from build123d import *

# Parameters (mm, degrees)
SKETCH1_W               = 52
SKETCH1_H               = 107
SKETCH1_R               = 3.25
BOSS_EXTRUDE1_DEPTH     = 3
SKETCH2_W               = 3
SKETCH2_H               = 35
BOSS_EXTRUDE2_DEPTH     = 35
SKETCH3_W               = 52
SKETCH3_H               = 5
BOSS_EXTRUDE3_DEPTH     = 25
SKETCH4_R               = 7.5
CUT_EXTRUDE1_DEPTH      = 71.585055075
CUT_EXTRUDE2_DEPTH      = 111.927904515
CUT_EXTRUDE2_DEPTH_BACK = 111.927904515
SKETCH5_W               = 35
SKETCH5_H               = 7


with BuildPart() as part:
    # Sketch1 → Boss-Extrude1 (new body)
    with BuildSketch(Plane(origin=(0, 0, 0), x_dir=(1, 0, 0), z_dir=(0, 1, 0))):
        Rectangle(SKETCH1_W, SKETCH1_H)
        with Locations(Location((17.5, -12, 0), (0, 0, 270))):
            Circle(SKETCH1_R, mode=Mode.SUBTRACT)
    extrude(amount=BOSS_EXTRUDE1_DEPTH)

    # Sketch2 → Boss-Extrude2 (add)
    with BuildSketch(Plane.XZ):
        with Locations((-24.5, 0)):
            Rectangle(SKETCH2_W, SKETCH2_H)
        with Locations((24.5, 0)):
            Rectangle(SKETCH2_W, SKETCH2_H)
    extrude(amount=BOSS_EXTRUDE2_DEPTH)

    # Sketch3 → Boss-Extrude3 (add)
    with BuildSketch(Plane.XZ):
        with Locations((0, 46)):
            Rectangle(SKETCH3_W, SKETCH3_H)
        with Locations((0, -46)):
            Rectangle(SKETCH3_W, SKETCH3_H)
    extrude(amount=BOSS_EXTRUDE3_DEPTH)

    # Sketch4 → Cut-Extrude1 (cut, through all)
    with BuildSketch(Plane(origin=(0, 3, 0), x_dir=(1, 0, 0), z_dir=(0, 1, 0))):
        with Locations(Location((0, 20, 0), (0, 0, 270))):
            Circle(SKETCH4_R)
    extrude(amount=-CUT_EXTRUDE1_DEPTH, mode=Mode.SUBTRACT)

    # Sketch5 → Cut-Extrude2 (cut, two sides: drawn at the far end of the back side and taken through both)
    with BuildSketch(Plane(origin=(0, 0, -48.5), x_dir=(-1, 0, 0), z_dir=(0, 0, -1)).offset(-CUT_EXTRUDE2_DEPTH_BACK)):
        with Locations((0, -10.5)):
            Rectangle(SKETCH5_W, SKETCH5_H)
    extrude(amount=CUT_EXTRUDE2_DEPTH + CUT_EXTRUDE2_DEPTH_BACK, mode=Mode.SUBTRACT)


solid = part.part
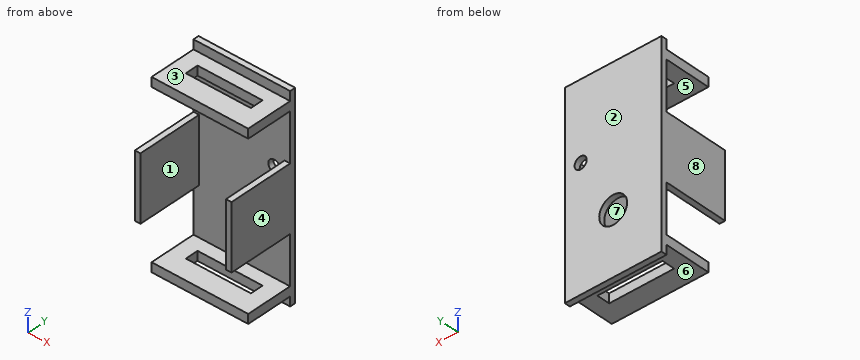
Verification items for the finished model (mm, model axes). Face numbers are marked on the shaded views. A direction names the side the tool comes from. Coordinates: 2 decimals unless noted, no trailing zeros. Order: outer loops, then holes, each group sorted by start corner. A loop starts at its lowest first (then second) coordinate and runs counter-clockwise, first axis right, second up. Notation, with made-up numbers: (74.5, 52) -> (91.5, 52) arc R12 cw to (91.5, 75) -> close; hole circle Ø11 at (55, 62.5). An arc over 180 degrees is marked (long way). Put each result on its own line as item: value. Start each with the question number.
1. Cross-section at D-D, the plane y = -2. Record the boundary of the cut face in (x, z).
2. Cross-section at A-A, the plane y = -13. Record the boundary of the cut face in (x, z).
3. Material ranges on L1, parallel to Z at x = -24, y = -4; L2, parallel to X at y = -28.5, z = -8.5; L3, parallel to Z at x = -2.5, y = -18.5, recorded low to high. Write a range as [from, to].
4. Cross-section at B-B, the plane z = 12. Record the boundary of the cut face in (x, y).
5. Mould release check, pull along X, two halves, no side actions. Record for the marked faces 6, 7 and 8: released by +X, released by -X, zero draft, split by the parting line, or undercut.
6. Go/stop test with flat-tipped pins: pin 1 Ø12.5 at (x, y) = (-9.5, -13) entering from -Z; pin 2 Ø2 at (x, y) = (0.5, -9.5) entering from -Z; pin 3 Ø5.5 at (x, z) = (-5, 45) entering from -Y; pin 4 Ø2 at (x, z) = (-10.5, -18) entering from -Y. Record where each tip stops, or that it passes through.
7. Cross-section at C-C, the plane x = 4.5. Record the boundary of the cut face in (y, z), then the cut area to 3 significant figures.
8. Access from +Z, -Z, +X, -X, +Y, -Y to the whole of each face (thin tool, end or side, straight path). Record for the marked faces 1, 2, 3, 4 and 5.
Computed:
1. outline: (-26, -48.5) -> (26, -48.5) -> (26, -43.5) -> (-26, -43.5) -> close; (-26, -17.5) -> (-23, -17.5) -> (-23, 17.5) -> (-26, 17.5) -> close; (-26, 43.5) -> (26, 43.5) -> (26, 48.5) -> (-26, 48.5) -> close; (23, -17.5) -> (26, -17.5) -> (26, 17.5) -> (23, 17.5) -> close
2. outline: (-26, -48.5) -> (-17.5, -48.5) -> (-17.5, -43.5) -> (-26, -43.5) -> close; (-26, -17.5) -> (-23, -17.5) -> (-23, 17.5) -> (-26, 17.5) -> close; (-26, 43.5) -> (-17.5, 43.5) -> (-17.5, 48.5) -> (-26, 48.5) -> close; (17.5, -48.5) -> (26, -48.5) -> (26, -43.5) -> (17.5, -43.5) -> close; (17.5, 43.5) -> (26, 43.5) -> (26, 48.5) -> (17.5, 48.5) -> close; (23, -17.5) -> (26, -17.5) -> (26, 17.5) -> (23, 17.5) -> close
3. L1: [-48.5, -43.5], [-17.5, 17.5], [43.5, 48.5]
3. L2: [-26, -23], [23, 26]
3. L3: [-48.5, -43.5], [43.5, 48.5]
4. outline: (-26, -35) -> (-23, -35) -> (-23, 0) -> (14.25, 0) -> (14.25, 3) -> (-26, 3) -> close; (20.75, 0) -> (23, 0) -> (23, -35) -> (26, -35) -> (26, 3) -> (20.75, 3) -> close
5. face 6: zero draft
5. face 7: undercut
5. face 8: released by -X
6. pin 1: z = -48.5
6. pin 2: through
6. pin 3: y = -25
6. pin 4: y = 0
7. outline: (-25, -48.5) -> (-14, -48.5) -> (-14, -43.5) -> (-25, -43.5) -> close; (-25, 43.5) -> (-14, 43.5) -> (-14, 48.5) -> (-25, 48.5) -> close; (-7, -48.5) -> (0, -48.5) -> (0, -53.5) -> (3, -53.5) -> (3, -26) -> (0, -26) -> (0, -43.5) -> (-7, -43.5) -> close; (-7, 43.5) -> (0, 43.5) -> (0, -14) -> (3, -14) -> (3, 53.5) -> (0, 53.5) -> (0, 48.5) -> (-7, 48.5) -> close
7. area: 465 mm2
8. face 1: -Y
8. face 2: +Z, -Z, +X, -X, +Y
8. face 3: +Z, +X, -X, -Y
8. face 4: +Z, -Z, +X, +Y, -Y
8. face 5: +X, -X, -Y
